For this review, take the finished solid that the model builds, in its own axes (mm). A direction names the side the tool comes from. Coordinates: 2 decimals unless noted, no trailing zeros. Write each loop counter-clockwise with the first axis right and the second up, starting at its lowest first coordinate (ties: lowest second). Pieces come first, ordered by that corner, then holes.
Autodesk Inventor part; units mm, degrees
ref_plane "YZ Plane" through (0, 0, 0) normal (1, 0, 0) x (0, 1, 0)
ref_plane "XZ Plane" through (0, 0, 0) normal (0, 1, 0) x (-1, 0, 0)
ref_plane "XY Plane" through (0, 0, 0) normal (0, 0, 1) x (1, 0, 0)
sketch "Boceto1" plane through (0, 0, 0) normal (0, 1, 0) x (-1, 0, 0)
  line L0 (15, 34.35) -> (15, -34.35)
  line L1 (15, -34.35) -> (-15, -34.35)
  line L2 (-15, -34.35) -> (-15, 34.35)
  line L3 (-15, 34.35) -> (15, 34.35)
  line L4 (15, 34.35) -> (-15, -34.35) construction
  line L5 (15, -34.35) -> (-15, 34.35) construction
  point P0 (0, 0)
  dimension "d0" = 68.7
  dimension "d1" = 30
extrude "Extrusión1" add sketch "Boceto1" along normal blind 32
sketch "Boceto2" plane through (-15, 0, 34.35) normal (0, 0, 1) x (1, 0, 0)
  line L0 (0, 32) -> (30, 32)
  line L1 (30, 32) -> (95.8937, -60.4136)
  line L2 (30, 32) -> (143.5, 32) construction
  line L3 (95.8937, -60.4136) -> (71.4672, -77.8304)
  line L4 (71.4672, -77.8304) -> (5.5735, 14.5832)
  line L5 (5.5735, 14.5832) -> (30, 32)
  point P0 (15, 0)
  dimension "d4" = 113.5
  dimension "d5" = 54.51
  dimension "d6" = 30
  dimension "d7" = 90
extrude "Extrusión2" add sketch "Boceto2" along normal blind 7
sketch "Boceto3" plane through (15, 0, -34.35) normal (0, 0, -1) x (-1, 0, 0)
  line L0 (0, 32) -> (-65.8937, -60.4136)
  line L1 (-41.4672, -77.8304) -> (14.0283, 0)
  line L2 (-65.8937, -60.4136) -> (-41.4672, -77.8304)
  line L3 (0, 32) -> (24.4265, 14.5832)
  line L4 (0, 32) -> (-65.8937, -60.4136)
  line L5 (-41.4672, -77.8304) -> (-65.8937, -60.4136)
  line L6 (-41.4672, -77.8304) -> (24.4265, 14.5832)
  line L7 (24.4265, 14.5832) -> (0, 32)
  point P0 (15, 0)
extrude "Extrusión3" add sketch "Boceto3" along normal blind 7
sketch "Boceto4" plane through (0, 0, 0) normal (0, 0, 1) x (1, 0, 0)
  line L0 (15, 32) -> (-15, 32)
  line L1 (-15, 32) -> (-82.3451, -62.4492)
  line L2 (-15, 32) -> (101, 32) construction
  line L3 (-82.3451, -62.4492) -> (-72.5745, -69.4159)
  line L4 (-72.5745, -69.4159) -> (-15, 11.3303)
  line L5 (-15, 0) -> (-15, 32)
  line L6 (-15, 11.3303) -> (-15, 32)
  point P0 (0, 0)
  dimension "d12" = 116
  dimension "d13" = 125.49
  dimension "d14" = 12
extrude "Extrusión4" add sketch "Boceto4" along normal blind 12
properties part number "structure"
Q1. Tool access review of faces 1 (the flat face through (15, 16, 0)), 2 (the flat face through (2.958, 23.414, -37.801)), 3 (the flat face through (2.616, 23.17, 37.801)), 4 (the flat face through (-7, 19, -34.35)), 5 (the flat face through (0, 0, 0)): name each direction out of +Z, -Z, +X, -X, +Y, -Y from which nothing blocks a thin tool from reaching the whole face with its end or side.
Ans:
face 1: +X, +Y, -Y
face 2: -Z, -X, +Y
face 3: +Z, -X, +Y
face 4: -Z, -X
face 5: +X, -Y
Q2. Add section C-C (x = -7). State the section outline as (y, z) points, then the cut area to 3 significant figures.
Ans:
outline: (0, -34.35) - (11.18, -34.35) - (11.18, -41.35) - (16.31, -41.35) - (16.31, -34.35) - (32, -34.35) - (32, 34.35) - (16.31, 34.35) - (16.31, 41.35) - (11.18, 41.35) - (11.18, 34.35) - (0, 34.35) - close
area: 2,270 mm2
Q3. Add section B-B (x = 28.5). State the section outline as (y, z) points.
Ans:
outline: (-38.61, -41.35) - (13.07, -41.35) - (13.07, -34.35) - (-38.61, -34.35) - close; (-38.61, 34.35) - (13.07, 34.35) - (13.07, 41.35) - (-38.61, 41.35) - close
Q4. Add section A-A (y = -8). State the section outline as (x, z) points.
Ans:
outline: (-43.52, 0) - (-28.78, 0) - (-28.78, 12) - (-43.52, 12) - close; (6.68, -41.35) - (43.52, -41.35) - (43.52, -34.35) - (6.68, -34.35) - close; (6.68, 34.35) - (43.52, 34.35) - (43.52, 41.35) - (6.68, 41.35) - close
Q5. Add section D-D (z = -32). State the section outline as (x, y) points, then the cut area to 3 significant figures.
Ans:
outline: (-15, 0) - (15, 0) - (15, 32) - (-15, 32) - close
area: 960 mm2
Q6. For probe 1 along Z at (x, y) = (58.5, -64); probe 2 along X at (y, z) = (18.5, 21.5); probe 3 along Y at (x, z) = (-1, 10.5), list the stretches that pass through material, from the lowest coordinate up.
Ans:
probe 1: z = -41.35 to -34.35, 34.35 to 41.35
probe 2: x = -15 to 15
probe 3: y = 0 to 32
Q7. Clearance check with flat-ended pins moving along their axes: pin 1 Ø9.5 at (y, z) = (22.5, 8.5) entering from +X; pin 2 Ø15 at (x, y) = (-6, 9.5) entering from +Z; pin 3 Ø2 at (y, z) = (6.5, 23) entering from -X; pin 4 Ø1 at (y, z) = (-52, 9) entering from -X. State where each tip first meets the part, or that it passes through.
Ans:
pin 1: stops at x = 15
pin 2: stops at z = 41.35
pin 3: stops at x = -15
pin 4: stops at x = -75.25
Q8. Draft analysis for pull direction Z (two halves, no side actions). For faces 6 (the flat face through (47.486, -13.56, 37.801)), 7 (the flat face through (-6, 19, 34.35)), 8 (the flat face through (44, -31, -34.35)), 9 (the flat face through (36, -27, -41.35)), state which applies: +Z half, -Z half, draft (parallel to the pull), parting line (faces both ways), or undercut.
Ans:
face 6: draft
face 7: +Z half
face 8: undercut
face 9: -Z half
